```python
from build123d import *

# Parameters (mm, degrees)
SKETCH1_R                                      = 8.75
SKETCH1_R_2                                    = 1
BOSS_EXTRUDE1_DEPTH                            = 1.5
CBORE_FOR_0_SOCKET_HEAD_CAP_SCREW2_D           = 1.778
CBORE_FOR_0_SOCKET_HEAD_CAP_SCREW2_DEPTH       = 7.5
CBORE_FOR_0_SOCKET_HEAD_CAP_SCREW2_CBORE_D     = 3.175
CBORE_FOR_0_SOCKET_HEAD_CAP_SCREW2_CBORE_DEPTH = 1.016
CBORE_FOR_0_SOCKET_HEAD_CAP_SCREW2_TIP         = 0.53416509


with BuildPart() as part:
    # Sketch1 → Boss-Extrude1 (new body)
    with BuildSketch(Plane(origin=(0, 0, 0), x_dir=(1, 0, 0), z_dir=(0, 1, 0))):
        with BuildLine():
            Line((-3, -12.1346611), (-3, -12.5))
            ThreePointArc((-3, -12.5), (0, -15.5), (3, -12.5))
            Line((3, -12.5), (3, -12.1346611))
            ThreePointArc((3, -12.1346611), (6.25, -10.825317547), (9.008924778, -8.665406761))
            Line((9.008924778, -8.665406761), (9.325317547, -8.848076211))
            ThreePointArc((9.325317547, -8.848076211), (13.423393759, -7.75), (12.325317547, -3.651923789))
            Line((12.325317547, -3.651923789), (12.008924778, -3.469254338))
            ThreePointArc((12.008924778, -3.469254338), (12.5, 0), (12.008924778, 3.469254338))
            Line((12.008924778, 3.469254338), (12.325317547, 3.651923789))
            ThreePointArc((12.325317547, 3.651923789), (13.423393759, 7.75), (9.325317547, 8.848076211))
            Line((9.325317547, 8.848076211), (9.008924778, 8.665406761))
            ThreePointArc((9.008924778, 8.665406761), (6.25, 10.825317547), (3, 12.1346611))
            Line((3, 12.1346611), (3, 12.5))
            ThreePointArc((3, 12.5), (0, 15.5), (-3, 12.5))
            Line((-3, 12.5), (-3, 12.1346611))
            ThreePointArc((-3, 12.1346611), (-6.25, 10.825317547), (-9.008924778, 8.665406761))
            Line((-9.008924778, 8.665406761), (-9.325317547, 8.848076211))
            ThreePointArc((-9.325317547, 8.848076211), (-13.423393759, 7.75), (-12.325317547, 3.651923789))
            Line((-12.325317547, 3.651923789), (-12.008924778, 3.469254338))
            ThreePointArc((-12.008924778, 3.469254338), (-12.5, 0), (-12.008924778, -3.469254338))
            Line((-12.008924778, -3.469254338), (-12.325317547, -3.651923789))
            ThreePointArc((-12.325317547, -3.651923789), (-13.423393759, -7.75), (-9.325317547, -8.848076211))
            Line((-9.325317547, -8.848076211), (-9.008924778, -8.665406761))
            ThreePointArc((-9.008924778, -8.665406761), (-6.25, -10.825317547), (-3, -12.1346611))
        make_face()
        with Locations(Location((0, 0, 0), (0, 0, 270))):
            Circle(SKETCH1_R, mode=Mode.SUBTRACT)
        with Locations(Location((-10.825317547, 6.25, 0), (0, 0, 270))):
            Circle(SKETCH1_R_2, mode=Mode.SUBTRACT)
        with Locations(Location((10.825317547, 6.25, 0), (0, 0, 270))):
            Circle(SKETCH1_R_2, mode=Mode.SUBTRACT)
        with Locations(Location((0, -12.5, 0), (0, 0, 270))):
            Circle(SKETCH1_R_2, mode=Mode.SUBTRACT)
    extrude(amount=BOSS_EXTRUDE1_DEPTH)

    # CBORE for #0 Socket Head Cap Screw2
    with Locations(Plane(origin=(-10.825317547, 1.5, 6.25), x_dir=(0, 0, 1), z_dir=(0, 1, 0))):
        with Locations((0, 0), (-18.75, 10.825317547), (0, 21.650635094)):
            CounterBoreHole(CBORE_FOR_0_SOCKET_HEAD_CAP_SCREW2_D / 2, CBORE_FOR_0_SOCKET_HEAD_CAP_SCREW2_CBORE_D / 2, CBORE_FOR_0_SOCKET_HEAD_CAP_SCREW2_CBORE_DEPTH, depth=CBORE_FOR_0_SOCKET_HEAD_CAP_SCREW2_DEPTH)
            with Locations((0, 0, -(CBORE_FOR_0_SOCKET_HEAD_CAP_SCREW2_DEPTH + CBORE_FOR_0_SOCKET_HEAD_CAP_SCREW2_TIP / 2))):  # 118° drill point
                Cone(0, CBORE_FOR_0_SOCKET_HEAD_CAP_SCREW2_D / 2, CBORE_FOR_0_SOCKET_HEAD_CAP_SCREW2_TIP, mode=Mode.SUBTRACT)


solid = part.part
```
The listing builds one solid part. Answer for the finished solid, in the listing's coordinates (mm). A direction names the side the tool comes from. Coordinates: 2 decimals unless noted, no trailing zeros. Write each loop counter-clockwise with the first axis right and the second up, starting at its lowest first coordinate (ties: lowest second). Pieces come first, ordered by that corner, then holes.
Q1. Section C-C, the plane y = 0.85 is taken. Give the number of separate pieces and of enclosed holes in the cut face, then the cut area to 3 significant figures.
Returned:
separate pieces: 1
enclosed holes: 7
area: 306 mm2
Q2. Section D-D, the plane z = 6.25 is taken. Write down the section's boundary in (x, y).
Returned:
outline: (-13.83, 0) - (-11.71, 0) - (-11.71, 0.48) - (-12.41, 0.48) - (-12.41, 1.5) - (-13.83, 1.5) - close; (-9.94, 0) - (-6.12, 0) - (-6.12, 1.5) - (-9.24, 1.5) - (-9.24, 0.48) - (-9.94, 0.48) - close; (6.12, 0) - (9.94, 0) - (9.94, 0.48) - (9.24, 0.48) - (9.24, 1.5) - (6.12, 1.5) - close; (11.71, 0) - (13.83, 0) - (13.83, 1.5) - (12.41, 1.5) - (12.41, 0.48) - (11.71, 0.48) - close
Q3. Given P1, Ø10.5, axis at x = 0, z = 0, coming from the -Y side; P2, Ø2.5, axis at x = 10.83, z = 6.25, coming from the +Y side, each flat-ended and moving along its own axis, determine where each tip first touches the part or whether it passes through.
Returned:
P1: passes through
P2: stops at y = 0.48
Q4. Find the intervals of material crossed by line 1 along Z through (x, y) = (10.25, 1); line 2 along X through (y, z) = (1.45, -7); line 3 along X through (y, z) = (0.75, 7), in increasing order.
Returned:
line 1: z = -9.19 to -7.07, -5.43 to 4.77, 7.73 to 9.19
line 2: x = -13.73 to -11.49, -10.16 to -5.25, 5.25 to 10.16, 11.49 to 13.73
line 3: x = -13.73 to -12.22, -9.43 to -5.25, 5.25 to 9.43, 12.22 to 13.73
Q5. The mould has two halves that part along X. Classify faces 3 (the cylindrical face through (12.5, 0.7, 0)), 4 (the flat face through (9, 0, 0)), 5 (the cylindrical face through (-0.6, 0.7, 11.7)): released by +X, released by -X, zero draft, split by the parting line, or undercut.
Returned:
face 3: released by +X
face 4: zero draft
face 5: undercut
Q6. Section A-A, the plane z = 0 is taken. Write down the section's boundary in (x, y).
Returned:
outline: (-12.5, 0) - (-8.75, 0) - (-8.75, 1.5) - (-12.5, 1.5) - close; (8.75, 0) - (12.5, 0) - (12.5, 1.5) - (8.75, 1.5) - close
Q7. Which of the six approach directions +Z, -Z, +X, -X, +Y, -Y give full straight-line access (tool end or side, diameter ignored) to faces 1 (the cylindrical face through (-9.25, 1, 6.04)), 2 (the cylindrical face through (-12.5, 0.7, 0))?
Returned:
face 1: +Y
face 2: -X, +Y, -Y
Q8. Section B-B, the plane x = 0 is taken. Write down the section's boundary in (y, z), then the cut area to 3 significant figures.
Returned:
outline: (0, -15.5) - (1.5, -15.5) - (1.5, -14.09) - (0.48, -14.09) - (0.48, -13.39) - (0, -13.39) - close; (0, -11.61) - (0.48, -11.61) - (0.48, -10.91) - (1.5, -10.91) - (1.5, -8.75) - (0, -8.75) - close; (0, 8.75) - (1.5, 8.75) - (1.5, 11.5) - (0, 11.5) - close; (0, 13.5) - (1.5, 13.5) - (1.5, 15.5) - (0, 15.5) - close
area: 13.2 mm2
